```python
from build123d import *

# Parameters (mm, degrees)
F0_W      = 25
F0_H      = 35
F1_DEPTH  = 4
F2_R      = 1.675
F3_DEPTH  = 25
F4_W      = 25
F4_H      = 11
F5_DEPTH  = 13
F7_DEPTH  = 6
F8_R      = 8
F9_DEPTH  = 6
F2_R_2    = 3
F10_DEPTH = 2
F11_R     = 5
F13_DEPTH = 2
F14_W     = 11
F14_H     = 17
F15_DEPTH = 2
F16_R     = 1.45
F17_DEPTH = 25
F18_R     = 5
F19_R     = 2


with BuildPart() as f1:
    # F0 (on Top) → F1 (new body)
    with BuildSketch(Plane.XY):
        with Locations((12.5, 17.5)):
            Rectangle(F0_W, F0_H)
    extrude(amount=F1_DEPTH)

    # F2 (on face) → F3 (cut)
    with BuildSketch(Plane.XY.offset(4)):
        with BuildLine():
            ThreePointArc((3.325, 18.5605346784), (5, 16.8855346784), (6.675, 18.5605346784))
            ThreePointArc((6.675, 18.5605346784), (5, 20.2355346784), (3.325, 18.5605346784))
        make_face()
        with Locations((20, 18.5605346784)):
            Circle(F2_R)
        with Locations((20, 3.5605346784)):
            Circle(F2_R)
        with Locations((5, 3.5605346784)):
            Circle(F2_R)
    extrude(amount=-F3_DEPTH, mode=Mode.SUBTRACT)

    # F4 (on face) → F5 (join)
    with BuildSketch(Plane.XY.offset(4)):
        with Locations((12.5, 29.5)):
            Rectangle(F4_W, F4_H)
    extrude(amount=F5_DEPTH)

    # F6 (on face) → F7 (cut)
    with BuildSketch(Plane(origin=(0, 35, 0), x_dir=(-1, 0, 0), z_dir=(0, 1, 0))):
        with BuildLine():
            ThreePointArc((-18.5, 17), (-12.5, 11), (-6.5, 17))
            Line((-6.5, 17), (-18.5, 17))
        make_face()
    extrude(amount=-F7_DEPTH, mode=Mode.SUBTRACT)

    # F8 (on face) → F9 (cut)
    with BuildSketch(Plane.XZ.offset(-24)):
        with Locations((12.5, 17)):
            Circle(F8_R)
    extrude(amount=-F9_DEPTH, mode=Mode.SUBTRACT)

    # F2 (on face) → F10 (cut)
    with BuildSketch(Plane.XY.offset(4)):
        with BuildLine():
            ThreePointArc((8, 18.5605346784), (5, 21.5605346784), (2, 18.5605346784))
            ThreePointArc((2, 18.5605346784), (5, 15.5605346784), (8, 18.5605346784))
        make_face()
        with BuildLine():
            ThreePointArc((3.325, 18.5605346784), (5, 20.2355346784), (6.675, 18.5605346784))
            ThreePointArc((6.675, 18.5605346784), (5, 16.8855346784), (3.325, 18.5605346784))
        make_face(mode=Mode.SUBTRACT)
        with Locations((20, 18.5605346784)):
            Circle(F2_R_2)
        with Locations((20, 18.5605346784)):
            Circle(F2_R, mode=Mode.SUBTRACT)
        with Locations((20, 3.5605346784)):
            Circle(F2_R_2)
        with Locations((20, 3.5605346784)):
            Circle(F2_R, mode=Mode.SUBTRACT)
        with Locations((5, 3.5605346784)):
            Circle(F2_R_2)
        with Locations((5, 3.5605346784)):
            Circle(F2_R, mode=Mode.SUBTRACT)
    extrude(amount=-F10_DEPTH, mode=Mode.SUBTRACT)

    # F11
    f11_edges = [f1.edges().sort_by_distance(p)[0] for p in [
        (0, 0, 2),
        (25, 0, 2),
    ]]
    fillet(f11_edges, radius=F11_R)

    # F12 (on face) → F13 (join)
    with BuildSketch(Plane(origin=(0, 0, 0), x_dir=(0, -1, 0), z_dir=(-1, 0, 0))):
        Polygon((-35, 17), (-35, 0), (-24, 0), (-24, 4), (-24, 17), align=None)
    extrude(amount=F13_DEPTH)

    # F14 (on face) → F15 (join)
    with BuildSketch(Plane.YZ.offset(25)):
        with Locations((29.5, 8.5)):
            Rectangle(F14_W, F14_H)
    extrude(amount=F15_DEPTH)

    # F16 (on face) → F17 (cut)
    with BuildSketch(Plane.XY.offset(17)):
        with Locations((0.45, 30.55)):
            Circle(F16_R)
        with Locations((24.55, 30.55)):
            Circle(F16_R)
    extrude(amount=-F17_DEPTH, mode=Mode.SUBTRACT)

    # F18
    f18_edges = [f1.edges().sort_by_distance(p)[0] for p in [
        (-2, 24, 8.5),
        (-2, 35, 8.5),
        (27, 35, 8.5),
        (27, 24, 8.5),
    ]]
    fillet(f18_edges, radius=F18_R)

    # F19
    f19_edges = [f1.edges().sort_by_distance(p)[0] for p in [
        (12.5, 24, 4),
        (23.581139, 24.256584, 4),
        (1.418861, 24.256584, 4),
    ]]
    fillet(f19_edges, radius=F19_R)


solid = f1.part
```
Geometry: final body of the model. Coordinates: model frame, mm. A direction names the side the tool comes from. Round coordinates to 2 decimals unless told otherwise and drop trailing zeros. Order: outer loops, then holes, each group sorted by start corner. A loop starts at its lowest first (then second) coordinate and runs counter-clockwise, first axis right, second up. Notation, with made-up numbers: (78.25, 84.5) - (132.25, 84.5) arc R14 ccw to (132.25, 110.5) - close; hole circle Ø6 at (22, -19). An arc over 180 degrees is marked (long way). Write item = value, one per line. Start each with the question number.
Q1. Cut plane C-C on x = 5.75. Return the cut outline in (y, z).
Q2. Cut plane B-B on y = 33. Return the cut outline in (x, z).
Q3. Pin query (flat end, axial travel): pin 1 (7 mm diameter, centred on x = 10.5, y = 12.5, fed in from +Z); pin 2 (3 mm diameter, centred on y = 15, z = 1.5, fed in from -X); pin 3 (4 mm diameter, centred on x = 5, y = 3.56, fed in from -Z); pin 4 (9.5 mm diameter, centred on x = 5, y = 18.56, fed in from +Z). Return the tip coordinate at first contact, or that it passes through.
Q4. Access query for faces 4 (the flat face through (25, 15, 2)), 5 (the flat face through (0, 15, 2)), 6 (the flat face through (11, 30, 11)), 7 (the cylindrical face through (25, 25, 11)), 8 (the cylindrical face through (0, 25, 11)). Directions: +Z, -Z, +X, -X, +Y, -Y. A direction counts if a zero-diameter tool reaches every point of the face in a straight line with its end or side. Return the directions, or none.
Q5. Pull-direction query (Y, two-part tool) for faces 1 (the cylindrical face through (12.6, 32.5, 11)), 2 (the flat face through (12, 0, 2)), 3 (the cylindrical face through (4.35, 0.63, 3.01)); classes: +Y half, -Y half, draft (parallel to the pull), parting line (faces both ways), or undercut.
Q6. Cut plane D-D on x = 15.5. Return the cut outline in (y, z).
Q7. Ray query, line 1 (Y direction, x = 5, z = 0.45); line 2 (Y direction, x = 5, z = 3.5); line 3 (X direction, y = 20, z = 2.5). Return the intervals inside material, ascending. Write a range as from..to.
Q8. Cut plane A-A on z = 14.5. Return the cut outline in (x, y), and give its area (3 significant figures).
Outcome:
q1.outline = (0, 0) - (2.06, 0) - (2.06, 2) - (0.66, 2) - (0.66, 4) - (0, 4) - close; (5.06, 0) - (17.06, 0) - (17.06, 2) - (15.66, 2) - (15.66, 4) - (6.47, 4) - (6.47, 2) - (5.06, 2) - close; (20.06, 0) - (35, 0) - (35, 17) - (30, 17) - (30, 12.71) - (24, 12.71) - (24, 6) arc R2 cw to (22, 4) - (21.47, 4) - (21.47, 2) - (20.06, 2) - close
q2.outline = (-1, 0) - (26, 0) - (26, 17) - (18.5, 17) arc R6 cw to (6.5, 17) - (-1, 17) - close
q3.pin_1 = 4
q3.pin_2 = 0
q3.pin_3 = 0
q3.pin_4 = 4.49
q4.face_4 = +Z, -Z, +X, -Y
q4.face_5 = +Z, -Z, -X, -Y
q4.face_6 = +Z, -Y
q4.face_7 = +Z, +X, -Y
q4.face_8 = +Z, -X, -Y
q5.face_1 = draft
q5.face_2 = -Y half
q5.face_3 = undercut
q6.outline = (0, 0) - (35, 0) - (35, 11.8) - (30, 11.8) - (30, 9.58) - (24, 9.58) - (24, 6) arc R2 cw to (22, 4) - (0, 4) - close
q7.line_1 = 0..1.89, 5.24..16.89, 20.24..35
q7.line_2 = 0..0.56, 6.56..15.56, 21.56..35
q7.line_3 = 0..2.37, 7.63..17.37, 22.63..25
q8.outline = (-2, 29) arc R5 ccw to (3, 24) - (4.9, 24) - (4.9, 30) - (7.05, 30) - (7.05, 35) - (3, 35) arc R5 ccw to (-2, 30) - close; (17.95, 30) - (20.1, 30) - (20.1, 24) - (22, 24) arc R5 ccw to (27, 29) - (27, 30) arc R5 ccw to (22, 35) - (17.95, 35) - close; hole circle Ø2.9 at (0.45, 30.55); hole circle Ø2.9 at (24.55, 30.55)
q8.area = 139 mm^2
